Could you check a few things on this model? Use its own coordinates, in mm. Face numbers are marked on the shaded views. A direction names the side the tool comes from. Give positions to 0.01 mm unless a question says otherwise; leave off trailing zeros. Loops run counter-clockwise (first coordinate to the right, second up) from the corner with the lowest first, then second, coordinate; pieces in that order, holes last. Notation, with made-up numbers: (14, 40) - (65, 40) arc R20 cw to (65, 51) - close; hole circle Ø9 at (18, -13). An arc over 180 degrees is marked (long way). Write each question's results on one line, items separated by ' | '. Start each with the question number.
1) I want a section at D-D, the plane y = 11.5. Write out the boundary of the cut face in (x, z), and give its area (3 significant figures).
2) If we mould it in two halves opening along Z, with no side actions, what happens to the marked faces 1, 2 and 3? For each: +Z half, -Z half, draft (parallel to the pull), parting line (faces both ways), or undercut.
3) I want a section at B-B, the plane x = -4.75. Write out the boundary of the cut face in (y, z).
4) I want a section at C-C, the plane z = 3.75. Write out the boundary of the cut face in (x, y), and give its area (3 significant figures).
5) I'm going to push flat-ended pins straight in: pin 1 (6 mm diameter, centred on x = -9.5, y = -9.5, fed in from -Z); pin 2 (1 mm diameter, centred on x = -9, y = 8, fed in from -Z); pin 3 (5 mm diameter, centred on x = 10, y = -10.5, fed in from -Z); pin 4 (7 mm diameter, centred on x = 6.93, z = 4, fed in from +Y). Where does each tip first touch, or does it pass through?
6) I want a section at A-A, the plane z = 0. Write out the boundary of the cut face in (x, y).
7) If I drill on probe 1 along Z at (x, y) = (-2, -6); probe 2 along X at (y, z) = (-4, 0.25); probe 3 along Z at (x, y) = (1, -8), over which ranges is the centre line in solid material (lowest first)? Write a range as [from, to].
8) On a 3-axis mill with a long thin cutter (end or side, diameter ignored), from which of +Z, -Z, +X, -X, +Y, -Y can I reach the whole of each face in a straight line? I mean the marked faces 4 and 5. Say none if no direction works.
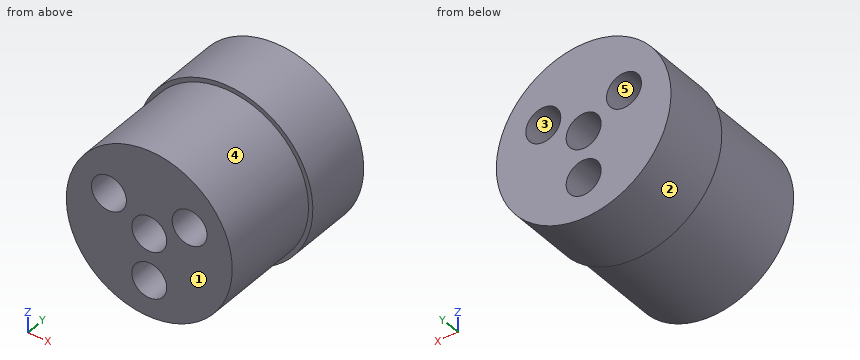
from build123d import *

# Parameters (mm, degrees)
SKETCH_1_R               = 14.25
EXTRUDE_1_DEPTH          = 15
HOLE_WIZARD_6_0_6_1_D    = 6
HOLE_WIZARD_6_0_6_2_D    = 6
PATTERN_CIRCULAR_1_COUNT = 3
SKETCH_6_R               = 15
SKETCH_6_R_2             = 14.25
EXTRUDE_2_DEPTH          = 12


with BuildPart() as part:
    # 스케치1 → 보스-돌출1 (new, symmetric)
    with BuildSketch(Plane(origin=(0, 0, 0), x_dir=(1, 0, 0), z_dir=(0, 1, 0))):
        with Locations(Location((0, 0, 0), (0, 0, 270))):
            Circle(SKETCH_1_R)
    extrude(amount=EXTRUDE_1_DEPTH, both=True)

    # Ø6.0 (6) 지름 구멍1 (through all)
    with Locations(Plane(origin=(0, 15, 0), x_dir=(1, 0, 0), z_dir=(0, 1, 0))):
        with Locations((0, 0)):
            Hole(HOLE_WIZARD_6_0_6_1_D / 2)

    # Ø6.0 (6) 지름 구멍2 (through all)
    with Locations(Plane(origin=(0, 15, 0), x_dir=(1, 0, 0), z_dir=(0, 1, 0))):
        with Locations((0, 8)):
            hole_wizard_6_0_6_2 = Hole(HOLE_WIZARD_6_0_6_2_D / 2)

    # 원형 패턴1: Ø6.0 (6) 지름 구멍2 ×3 about axis
    pattern_circular_1_axis = Axis((0, 0, 0), (0, 1, 0))
    for i in range(1, PATTERN_CIRCULAR_1_COUNT):
        add(hole_wizard_6_0_6_2.rotate(pattern_circular_1_axis, i * 360 / PATTERN_CIRCULAR_1_COUNT), mode=Mode.SUBTRACT)

    # 스케치6 → 보스-돌출2 (add)
    with BuildSketch(Plane(origin=(0, 15, 0), x_dir=(1, 0, 0), z_dir=(0, 1, 0))):
        with Locations(Location((0, 0, 0), (0, 0, 270))):
            Circle(SKETCH_6_R)
        with Locations(Location((0, 0, 0), (0, 0, 270))):
            Circle(SKETCH_6_R_2, mode=Mode.SUBTRACT)
    extrude(amount=-EXTRUDE_2_DEPTH)


solid = part.part
Answers:
1) outline: circle Ø30 at (0, 0); hole circle Ø6 at (-6.93, 4); hole circle Ø6 at (0, -8); hole circle Ø6 at (0, 0); hole circle Ø6 at (6.93, 4) | area: 594 mm2
2) face 1: draft | face 2: parting line | face 3: undercut
3) outline: (-15, -13.44) - (3, -13.44) - (3, -14.23) - (15, -14.23) - (15, 1.94) - (-15, 1.94) - close; (-15, 6.06) - (15, 6.06) - (15, 14.23) - (3, 14.23) - (3, 13.44) - (-15, 13.44) - close
4) outline: (-14.52, 3) - (-13.75, 3) - (-13.75, -15) - (-9.92, -15) - (-9.92, 15) - (-14.52, 15) - close; (-3.94, -15) - (3.94, -15) - (3.94, 15) - (-3.94, 15) - close; (9.92, -15) - (13.75, -15) - (13.75, 3) - (14.52, 3) - (14.52, 15) - (9.92, 15) - close | area: 485 mm2
5) pin 1: stops at z = -12.68 | pin 2: stops at z = -12.36 | pin 3: stops at z = -12.12 | pin 4: stops at y = 15
6) outline: (-15, 3) - (-14.25, 3) - (-14.25, -15) - (-3, -15) - (-3, 15) - (-15, 15) - close; (3, -15) - (14.25, -15) - (14.25, 3) - (15, 3) - (15, 15) - (3, 15) - close
7) probe 1: z = [-14.11, -10.24], [-5.76, -2.24], [2.24, 14.11] | probe 2: x = [-14.25, -2.99], [2.99, 14.25] | probe 3: z = [-14.21, -10.83], [-5.17, -2.83], [2.83, 14.21]
8) face 4: -Y | face 5: +Y, -Y
